from build123d import *

# Parameters (mm, degrees)
PAD_DEPTH         = 3
PAD001_DEPTH      = 6
SKETCH002_R       = 2
POCKET_DEPTH      = 6.001
POCKET_DEPTH_BACK = -0.001


with BuildPart() as horn:
    # Sketch → Pad (new body)
    with BuildSketch(Plane.XY):
        with BuildLine():
            ThreePointArc((-2.490104, -0.222222), (0, -2.5), (2.490104, -0.222222))
            Line((4.482187, 22.1), (2.490104, -0.222222))
            ThreePointArc((4.482187, 22.1), (4.5, 22.5), (4.482187, 22.9))
            Line((2.490104, 45.222222), (4.482187, 22.9))
            ThreePointArc((2.490104, 45.222222), (0, 47.5), (-2.490104, 45.222222))
            Line((-2.490104, 45.222222), (-4.482187, 22.9))
            ThreePointArc((-4.482187, 22.9), (-4.5, 22.5), (-4.482187, 22.1))
            Line((-4.482187, 22.1), (-2.490104, -0.222222))
        make_face()
    extrude(amount=-PAD_DEPTH)


with BuildPart() as cut:
    # Sketch001 → Pad001 (new body)
    with BuildSketch(Plane.XY):
        with BuildLine():
            ThreePointArc((-10, 0), (0, -10), (10, 0))
            Line((10, 0), (10, 70))
            ThreePointArc((10, 70), (0, 80), (-10, 70))
            Line((-10, 0), (-10, 70))
        make_face()
    extrude(amount=-PAD001_DEPTH)

    # Sketch002 → Pocket (cut, two sides)
    with BuildSketch(Plane.XY) as pocket_sk:
        with Locations((0, 70)):
            Circle(SKETCH002_R)
    extrude(amount=-POCKET_DEPTH, mode=Mode.SUBTRACT)
    extrude(pocket_sk.sketch, amount=-POCKET_DEPTH_BACK, mode=Mode.SUBTRACT)

    # Cut: cut Horn
    add(horn.part, mode=Mode.SUBTRACT)


solid = cut.part
The listing builds one solid part. Answer for the finished solid, in the listing's coordinates (mm). A direction names the side the tool comes from. Coordinates: 2 decimals unless noted, no trailing zeros. Order: outer loops, then holes, each group sorted by start corner. A loop starts at its lowest first (then second) coordinate and runs counter-clockwise, first axis right, second up.
Q1. A cutting plane is placed at B-B, the plane z = -2.2. Write down the section's boundary in (x, y), and give its area (3 significant figures).
Q2. Which of the six approach directions +Z, -Z, +X, -X, +Y, -Y give full straight-line access (tool end or side, diameter ignored) to faces 1 (the face through (0, -10, -3)), 2 (the face through (3.5, 11.1, -1.5))?
Q3. Given P1, Ø1.5, axis at x = 6, z = -3.5, coming from the -Y side; P2, Ø1, axis at x = 2, z = -4.5, coming from the +Y side, each flat-ended and moving along its own axis, determine where each tip first touches the part or whether it passes through.
Q4. A cutting plane is placed at D-D, the plane x = 8.5. Write down the section's boundary in (y, z).
Q5. Consider line 1 (Y direction, x = 0, z = -3.85); line 2 (Y direction, x = 0, z = -1.5); line 3 (Z direction, x = -3, y = 36.5). Determine where each line is inside the solid, lowest interval first.
Q6. A cutting plane is placed at C-C, the plane y = 13.5. Write down the section's boundary in (x, z), and give its area (3 significant figures).
Q7. A cutting plane is placed at A-A, the plane x = 0. Write down the section's boundary in (y, z).
Q8. For a pull along X with two mould halves and no side action, classify faces 3 (the face through (10, 35, -3)), 4 (the face through (0, 72, -3)), 5 (the face through (-10, 35, -3)) as pulls with the +X half, pulls with the -X half, needs draft (parallel to the pull), parting line crosses it, or undercut.
Answers follow:
1. outline: (-10, 0) arc R10 ccw to (10, 0) - (10, 70) arc R10 ccw to (-10, 70) - close; hole (-4.48, 22.1) - (-2.49, -0.22) arc R2.5 ccw to (2.49, -0.22) - (4.48, 22.1) arc R4.5 ccw to (4.48, 22.9) - (2.49, 45.22) arc R2.5 ccw to (-2.49, 45.22) - (-4.48, 22.9) arc R4.5 ccw to start; hole circle Ø4 at (0, 70)
1. area: 1,370 mm2
2. face 1: +Z, -Z, -Y
2. face 2: +Z
3. P1: stops at y = -8.51
3. P2: stops at y = 79.89
4. outline: (-5.27, -6) - (75.27, -6) - (75.27, 0) - (-5.27, 0) - close
5. line 1: y = -10 to 68, 72 to 80
5. line 2: y = -10 to -2.5, 47.5 to 68, 72 to 80
5. line 3: z = -6 to -3
6. outline: (-10, -6) - (10, -6) - (10, 0) - (3.71, 0) - (3.71, -3) - (-3.71, -3) - (-3.71, 0) - (-10, 0) - close
6. area: 97.7 mm2
7. outline: (-10, -6) - (68, -6) - (68, 0) - (47.5, 0) - (47.5, -3) - (-2.5, -3) - (-2.5, 0) - (-10, 0) - close; (72, -6) - (80, -6) - (80, 0) - (72, 0) - close
8. face 3: pulls with the +X half
8. face 4: undercut
8. face 5: pulls with the -X half
